Verification items for the finished model (mm, model axes). A direction names the side the tool comes from. Round coordinates to 2 decimals unless told otherwise and drop trailing zeros. Order: outer loops, then holes, each group sorted by start corner. A loop starts at its lowest first (then second) coordinate and runs counter-clockwise, first axis right, second up. Notation, with made-up numbers: (14, 6.25) -> (36, 6.25) arc R23 ccw to (36, 29.25) -> close; hole circle Ø6 at (-15.75, 46). An arc over 180 degrees is marked (long way). Return JSON: item names as keys, results as strings. Group by question number.
Item 1: Sectioned sample at C-C on y = 11.5. Record the cut outline in (x, z).
Item 2: Sectioned sample at A-A on x = 0. Record the cut outline in (y, z).
Item 3: Depth check by flat-ended pin: pin 1 Ø5.5 at (y, z) = (2.5, 12.5) entering from -X; pin 2 Ø2.5 at (y, z) = (3, 14.5) entering from +X; pin 3 Ø10 at (x, y) = (13, -0.5) entering from +Z; pin 4 Ø0.8 at (y, z) = (-7, 6) entering from +X. Enter the tip coordinate at first touch or a pass-through.
Item 4: Sectioned sample at D-D on z = 3.5. Record the cut outline in (x, y).
Item 5: Scan lines: probe 1 along Y at (x, z) = (0, 3.2); probe 2 along X at (y, z) = (1, 10.5); probe 3 along Y at (x, z) = (13, 17.5). Record each from-to range of solid material in increasing order. Write a range as from..to.
Item 6: Sectioned sample at B-B on z = 13.25. Record the cut outline in (x, y).
Item 7: Draft check along Y on faces 4 (the flat face through (-17.295, -12.115, 8.123)), 5 (the flat face through (14.44, 2.5, 21.63)), 6 (the flat face through (12.06, 8.84, 17.15)). Enter one of: pulls with the +Y half, pulls with the -Y half, needs draft (parallel to the pull), parting line crosses it, or undercut.
Item 8: Access from +Z, -Z, +X, -X, +Y, -Y to the whole of each face (thin tool, end or side, straight path). Record for faces 1 (the flat face through (-14.09, -17.16, 6.33)), 2 (the flat face through (-20.211, -6, 6)), 3 (the flat face through (-14, 5.08, 15)).
```python
from build123d import *

# Parameters (mm, degrees)
F0_R     = 25.4
F0_W     = 2.9527507722
F0_H     = 2.9527507722
F0_R_2   = 11.43
F0_W_2   = 2.8575006872
F0_H_2   = 2.8575006872
F0_W_3   = 4.0005007759
F0_H_3   = 4.0005007759
F1_DEPTH = 5.08
F2_DEPTH = 2.54
F3_DEPTH = 17.78
F0_W_4   = 2.54
F0_H_4   = 2.54
F0_W_5   = 2.5392780889
F0_H_5   = 2.5392780889
F4_DEPTH = 22.86
F5_DEPTH = 8.89
F6_SIZE  = 1.26999
F7_SIZE  = 2.032
F8_SIZE  = 1.27


# Not quite as in the source:
# - a fillet or chamfer is up to 0.001 mm smaller than in the source, because OpenCascade refuses the exact size


with BuildPart() as f1:
    # F0 (on Top) → F1 (new body)
    with BuildSketch(Plane.XY):
        Circle(F0_R)
        Polygon((-14.8460203377, -16.160586299), (-12.8199555069, -14.6287046778), (-11.2880738857, -16.6547695086), (-13.3141387165, -18.1866511298), align=None, mode=Mode.SUBTRACT)
        Polygon((-17.0199228451, -13.7883033603), (-18.4486722574, -10.9308026731), (-15.5911715701, -9.5020532608), (-14.1624221578, -12.359553948), align=None, mode=Mode.SUBTRACT)
        with Locations((-18.734421581, -5.5491779931)):
            Rectangle(F0_W, F0_H, mode=Mode.SUBTRACT)
        with Locations((0, -11.43)):
            Circle(F0_R_2, mode=Mode.SUBTRACT)
        with Locations((16.1819914356, -13.3789330721)):
            Rectangle(F0_W_2, F0_H_2, mode=Mode.SUBTRACT)
        with Locations((16.3652040064, -6.5969279967)):
            Rectangle(F0_W_3, F0_H_3, mode=Mode.SUBTRACT)
        Polygon((-10.1001541496, 17.7187103274), (-10.1592772274, 15.24), (10.1607219111, 15.24), (10.1607219111, 17.7792780889), (15.2392780889, 17.7792780889), (15.2392780889, 12.7007219111), (12.7, 12.7007219111), (12.7, 5.08), (15.24, 5.08), (15.24, 0), (10.16, 0), (10.16, 2.54), (-10.16, 2.54), (-10.16, 0), (-15.24, 0), (-15.24, 5.08), (-12.7, 5.08), (-12.7, 12.6992772274), (-15.2998458504, 12.7612896726), (-15.1787103274, 17.8398458504), align=None, mode=Mode.SUBTRACT)
    extrude(amount=F1_DEPTH)

    # F0 (on Top) → F2 (join)
    with BuildSketch(Plane.XY):
        with Locations((0, -11.43)):
            Circle(F0_R_2)
    extrude(amount=F2_DEPTH)

    # F0 (on Top) → F3 (join)
    with BuildSketch(Plane.XY):
        Polygon((10.1607219111, 15.24), (-10.1592772274, 15.24), (-10.2212896726, 12.6401541496), (-12.7, 12.6992772274), (-12.7, 5.08), (-10.16, 5.08), (-10.16, 2.54), (10.16, 2.54), (10.16, 5.08), (12.7, 5.08), (12.7, 12.7007219111), (10.1607219111, 12.7007219111), align=None)
    extrude(amount=F3_DEPTH)

    # F0 (on Top) → F4 (join)
    with BuildSketch(Plane.XY):
        Polygon((-10.1592772274, 15.24), (-12.7, 15.24), (-12.7, 12.6992772274), (-10.2212896726, 12.6401541496), align=None)
        Polygon((-12.7, 12.6992772274), (-12.7, 15.24), (-10.1592772274, 15.24), (-10.1001541496, 17.7187103274), (-15.1787103274, 17.8398458504), (-15.2998458504, 12.7612896726), align=None)
        with Locations((-11.43, 3.81)):
            Rectangle(F0_W_4, F0_H_4)
        Polygon((-12.7, 2.54), (-12.7, 5.08), (-15.24, 5.08), (-15.24, 0), (-10.16, 0), (-10.16, 2.54), align=None)
        with Locations((11.4303609556, 13.9703609556)):
            Rectangle(F0_W_5, F0_H_5)
        Polygon((10.1607219111, 17.7792780889), (10.1607219111, 15.24), (12.7, 15.24), (12.7, 12.7007219111), (15.2392780889, 12.7007219111), (15.2392780889, 17.7792780889), align=None)
        with Locations((11.43, 3.81)):
            Rectangle(F0_W_4, F0_H_4)
        Polygon((15.24, 5.08), (12.7, 5.08), (12.7, 2.54), (10.16, 2.54), (10.16, 0), (15.24, 0), align=None)
    extrude(amount=F4_DEPTH)

    # F0 (on Top) → F5 (join)
    with BuildSketch(Plane.XY):
        with Locations((-18.734421581, -5.5491779931)):
            Rectangle(F0_W, F0_H)
        Polygon((-15.5911715701, -9.5020532608), (-18.4486722574, -10.9308026731), (-17.0199228451, -13.7883033603), (-14.1624221578, -12.359553948), align=None)
        Polygon((-11.2880738857, -16.6547695086), (-12.8199555069, -14.6287046778), (-14.8460203377, -16.160586299), (-13.3141387165, -18.1866511298), align=None)
        with Locations((16.3652040064, -6.5969279967)):
            Rectangle(F0_W_3, F0_H_3)
        with Locations((16.1819914356, -13.3789330721)):
            Rectangle(F0_W_2, F0_H_2)
    extrude(amount=F5_DEPTH)

    # F6 (size 1.27 in the source; OpenCascade refuses exactly that, so slightly less here)
    f6_edges = [f1.edges().sort_by_distance(p)[0] for p in [
        (-18.734422, -4.072803, 8.89),
        (-20.210797, -5.549178, 8.89),
        (-18.734422, -7.025553, 8.89),
        (-17.258046, -5.549178, 8.89),
        (-17.019922, -10.216428, 8.89),
        (-17.734298, -12.359553, 8.89),
        (-15.591173, -13.073929, 8.89),
        (-14.876797, -10.930804, 8.89),
        (-12.301106, -17.42071, 8.89),
        (-12.054015, -15.641737, 8.89),
        (-13.832988, -15.394645, 8.89),
        (-14.08008, -17.173619, 8.89),
        (16.365204, -4.596678, 8.89),
        (14.364954, -6.596928, 8.89),
        (16.365204, -8.597178, 8.89),
        (18.365454, -6.596928, 8.89),
        (16.181991, -14.807683, 8.89),
        (17.610742, -13.378933, 8.89),
        (16.181991, -11.950183, 8.89),
        (14.753241, -13.378933, 8.89),
    ]]
    chamfer(f6_edges, length=F6_SIZE)

    # F7
    f7_edges = [f1.edges().sort_by_distance(p)[0] for p in [
        (-10.160722, 15.179432, 22.86),
        (-12.639432, 17.779278, 22.86),
        (-15.239278, 15.300568, 22.86),
        (-12.760568, 12.700722, 22.86),
        (-12.7, 5.08, 22.86),
        (-15.24, 2.54, 22.86),
        (-12.7, 0, 22.86),
        (-10.16, 2.54, 22.86),
        (12.7, 12.700722, 22.86),
        (15.239278, 15.24, 22.86),
        (12.7, 17.779278, 22.86),
        (10.160722, 15.24, 22.86),
        (10.16, 2.54, 22.86),
        (12.7, 0, 22.86),
        (15.24, 2.54, 22.86),
        (12.7, 5.08, 22.86),
    ]]
    chamfer(f7_edges, length=F7_SIZE)

    # F8
    f8_edges = [f1.edges().sort_by_distance(p)[0] for p in [
        (0, 2.54, 17.78),
        (0.000722, 15.24, 17.78),
        (-12.7, 8.889639, 17.78),
        (12.7, 8.890361, 17.78),
    ]]
    chamfer(f8_edges, length=F8_SIZE)


solid = f1.part
```
Recorded:
{
 "1": {"outline": "(-22.65, 0) -> (22.65, 0) -> (22.65, 5.08) -> (12.7, 5.08) -> (12.7, 16.51) -> (11.43, 17.78) -> (-11.43, 17.78) -> (-12.7, 16.51) -> (-12.7, 5.08) -> (-22.65, 5.08) -> close"},
 "2": {"outline": "(-25.4, 0) -> (25.4, 0) -> (25.4, 5.08) -> (15.24, 5.08) -> (15.24, 16.51) -> (13.97, 17.78) -> (3.81, 17.78) -> (2.54, 16.51) -> (2.54, 5.08) -> (0, 5.08) -> (0, 2.54) -> (-22.86, 2.54) -> (-22.86, 5.08) -> (-25.4, 5.08) -> close"},
 "3": {"pin 1": "x = -15.24", "pin 2": "x = 15.24", "pin 3": "z = 22.86", "pin 4": "x = 18.37"},
 "4": {"outline": "circle Ø50.8 at (0, 0); hole circle Ø22.86 at (0, -11.43)"},
 "5": {"probe 1": "-25.4..-22.86, 0..25.4", "probe 2": "-15.24..-10.16, 10.16..15.24", "probe 3": "0..5.08, 12.7..17.78"},
 "6": {"outline": "(-15.3, 12.76) -> (-12.7, 12.7) -> (-12.7, 5.08) -> (-15.24, 5.08) -> (-15.24, 0) -> (-10.16, 0) -> (-10.16, 2.54) -> (10.16, 2.54) -> (10.16, 0) -> (15.24, 0) -> (15.24, 5.08) -> (12.7, 5.08) -> (12.7, 12.7) -> (15.24, 12.7) -> (15.24, 17.78) -> (10.16, 17.78) -> (10.16, 15.24) -> (-10.16, 15.24) -> (-10.1, 17.72) -> (-15.18, 17.84) -> close"},
 "7": {"face 4": "pulls with the -Y half", "face 5": "needs draft", "face 6": "undercut"},
 "8": {"face 1": "+Z, -X, -Y", "face 2": "+Z, -X, +Y, -Y", "face 3": "+Z, -X"}
}
